Geometry check sheet. Reference: the model listing, model coordinates, mm. Face numbers are marked on the shaded views. Give positions to 0.01 mm unless a question says otherwise; leave off trailing zeros. Write each loop counter-clockwise with the first axis right and the second up, starting at its lowest first coordinate (ties: lowest second). Pieces come first, ordered by that corner, then holes. Notation, with made-up numbers: M -14,34.5 L -3,34.5 A18 ccw -3,52.5 Z; hole C 21,71.25 d6. An arc over 180 degrees is marked long. One line per item, written item: value. Start each with the question number.
1. Cross-section at C-C on x = -21. Record the cut outline in (y, z).
2. Cross-section at B-B on z = 4. Record the cut outline in (x, y).
3. Cross-section at A-A on y = -40. Record the cut outline in (x, z).
4. Release check for a two-part mould opening along X. For the marked faces 1 and 2 record: pulls with the +X half, pulls with the -X half, needs draft (parallel to the pull), parting line crosses it, or undercut.
5. Gauge pin test, flat ends, axial feed: pin 1 (4 mm diameter, centred on y = -30.5, z = -3, fed in from -X); pin 2 (2 mm diameter, centred on y = -20, z = 5, fed in from -X); pin 3 (1.5 mm diameter, centred on x = -23.5, y = -33.5, fed in from +Z). Record the tip position at first contact, or that the pin passes through.
6. Scan lines: line 1 (Z direction, x = 21, y = -9); line 2 (Z direction, x = -0.5, y = -42.5); line 3 (X direction, y = -23, z = -0.25). Record each from-to range of solid material in increasing order.
from build123d import *

# Parameters (mm, degrees)
F1_DEPTH = 48.26


# Not quite as in the source:
# - a feature names something its author has since deleted; it is built from what else it names


with BuildPart() as f1:
    # F0 (on Front) → F1 (new body)
    with BuildSketch(Plane.XZ):
        with BuildLine():
            ThreePointArc((3.556, -6.1591726717), (6.1591726717, -3.556), (7.112, 0))
            ThreePointArc((7.112, 0), (6.1591726717, 3.556), (3.556, 6.1591726717))
            ThreePointArc((3.556, 6.1591726717), (0, 7.112), (-3.556, 6.1591726717))
            ThreePointArc((-3.556, 6.1591726717), (-6.1591726717, 3.556), (-7.112, 0))
            ThreePointArc((-7.112, 0), (-6.1591726717, -3.556), (-3.556, -6.1591726717))
            ThreePointArc((-3.556, -6.1591726717), (0, -7.112), (3.556, -6.1591726717))
        make_face()
        with BuildLine():
            ThreePointArc((-10.668, -6.1591726717), (-8.0648273283, -3.556), (-7.112, 0))
            ThreePointArc((-7.112, 0), (-8.0648273283, 3.556), (-10.668, 6.1591726717))
            ThreePointArc((-10.668, 6.1591726717), (-14.224, 7.112), (-17.78, 6.1591726717))
            ThreePointArc((-17.78, 6.1591726717), (-20.3831726717, 3.556), (-21.336, 0))
            ThreePointArc((-21.336, 0), (-20.3831726717, -3.556), (-17.78, -6.1591726717))
            ThreePointArc((-17.78, -6.1591726717), (-14.224, -7.112), (-10.668, -6.1591726717))
        make_face()
        with BuildLine():
            ThreePointArc((-24.892, -6.1591726717), (-22.2888273283, -3.556), (-21.336, 0))
            ThreePointArc((-21.336, 0), (-22.2888273283, 3.556), (-24.892, 6.1591726717))
            ThreePointArc((-24.892, 6.1591726717), (-35.56, 0), (-24.892, -6.1591726717))
        make_face()
        with BuildLine():
            ThreePointArc((10.668, 6.1591726717), (8.0648273283, 3.556), (7.112, 0))
            ThreePointArc((7.112, 0), (8.0648273283, -3.556), (10.668, -6.1591726717))
            ThreePointArc((10.668, -6.1591726717), (14.224, -7.112), (17.78, -6.1591726717))
            ThreePointArc((17.78, -6.1591726717), (20.3831726717, -3.556), (21.336, 0))
            ThreePointArc((21.336, 0), (20.3831726717, 3.556), (17.78, 6.1591726717))
            ThreePointArc((17.78, 6.1591726717), (14.224, 7.112), (10.668, 6.1591726717))
        make_face()
        with BuildLine():
            ThreePointArc((24.892, 6.1591726717), (22.2888273283, 3.556), (21.336, 0))
            ThreePointArc((21.336, 0), (22.2888273283, -3.556), (24.892, -6.1591726717))
            ThreePointArc((24.892, -6.1591726717), (32.004, -6.1591726717), (35.56, 0))
            ThreePointArc((35.56, 0), (32.004, 6.1591726717), (24.892, 6.1591726717))
        make_face()
        with BuildLine():
            ThreePointArc((3.556, 6.1591726717), (6.1591726717, 3.556), (7.112, 0))
            ThreePointArc((7.112, 0), (8.0648273283, 3.556), (10.668, 6.1591726717))
            ThreePointArc((10.668, 6.1591726717), (7.112, 5.6520452644), (3.556, 6.1591726717))
        make_face()
        with BuildLine():
            ThreePointArc((24.892, 6.1591726717), (21.336, 5.6520452644), (17.78, 6.1591726717))
            ThreePointArc((17.78, 6.1591726717), (20.3831726717, 3.556), (21.336, 0))
            ThreePointArc((21.336, 0), (22.2888273283, 3.556), (24.892, 6.1591726717))
        make_face()
        with BuildLine():
            ThreePointArc((-7.112, 0), (-6.1591726717, 3.556), (-3.556, 6.1591726717))
            ThreePointArc((-3.556, 6.1591726717), (-7.112, 5.6520452644), (-10.668, 6.1591726717))
            ThreePointArc((-10.668, 6.1591726717), (-8.0648273283, 3.556), (-7.112, 0))
        make_face()
        with BuildLine():
            ThreePointArc((-21.336, 0), (-20.3831726717, 3.556), (-17.78, 6.1591726717))
            ThreePointArc((-17.78, 6.1591726717), (-21.336, 5.6520452644), (-24.892, 6.1591726717))
            ThreePointArc((-24.892, 6.1591726717), (-22.2888273283, 3.556), (-21.336, 0))
        make_face()
        with BuildLine():
            ThreePointArc((-24.892, -6.1591726717), (-21.336, -5.6520452644), (-17.78, -6.1591726717))
            ThreePointArc((-17.78, -6.1591726717), (-20.3831726717, -3.556), (-21.336, 0))
            ThreePointArc((-21.336, 0), (-22.2888273283, -3.556), (-24.892, -6.1591726717))
        make_face()
        with BuildLine():
            ThreePointArc((-10.668, -6.1591726717), (-7.112, -5.6520452644), (-3.556, -6.1591726717))
            ThreePointArc((-3.556, -6.1591726717), (-6.1591726717, -3.556), (-7.112, 0))
            ThreePointArc((-7.112, 0), (-8.0648273283, -3.556), (-10.668, -6.1591726717))
        make_face()
        with BuildLine():
            ThreePointArc((10.668, -6.1591726717), (8.0648273283, -3.556), (7.112, 0))
            ThreePointArc((7.112, 0), (6.1591726717, -3.556), (3.556, -6.1591726717))
            ThreePointArc((3.556, -6.1591726717), (7.112, -5.6520452644), (10.668, -6.1591726717))
        make_face()
        with BuildLine():
            ThreePointArc((21.336, 0), (20.3831726717, -3.556), (17.78, -6.1591726717))
            ThreePointArc((17.78, -6.1591726717), (21.336, -5.6520452644), (24.892, -6.1591726717))
            ThreePointArc((24.892, -6.1591726717), (22.2888273283, -3.556), (21.336, 0))
        make_face()
    extrude(amount=F1_DEPTH)


solid = f1.part
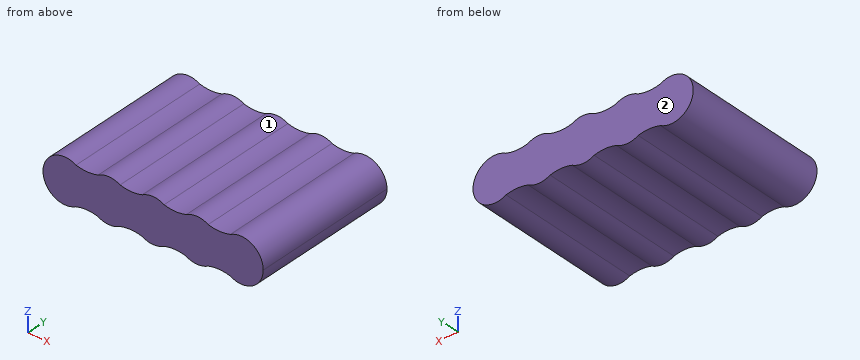
Report:
1. outline: M -48.26,-5.66 L 0,-5.66 L 0,5.66 L -48.26,5.66 Z
2. outline: M -34.33,-48.26 L 34.33,-48.26 L 34.33,0 L -34.33,0 Z
3. outline: M -24.89,-6.16 A12.72 cw -17.78,-6.16 A7.11 ccw -10.67,-6.16 A12.72 cw -3.56,-6.16 A7.11 ccw 3.56,-6.16 A12.72 cw 10.67,-6.16 A7.11 ccw 17.78,-6.16 A12.72 cw 24.89,-6.16 A7.11 ccw long 24.89,6.16 A12.72 cw 17.78,6.16 A7.11 ccw 10.67,6.16 A12.72 cw 3.56,6.16 A7.11 ccw -3.56,6.16 A12.72 cw -10.67,6.16 A7.11 ccw -17.78,6.16 A12.72 cw -24.89,6.16 A7.11 ccw long Z
4. face 1: undercut
4. face 2: needs draft
5. pin 1: stops at x = -35.49
5. pin 2: stops at x = -34.33
5. pin 3: stops at z = 5.99
6. line 1: z = -5.66 to 5.66
6. line 2: z = -7.09 to 7.09
6. line 3: x = -35.56 to 35.56
